Job drawing, mm, ordinate dimensions from the low corner. One solid piece. A direction names the side the tool comes from. Round coordinates to 2 decimals unless told otherwise and drop trailing zeros. Write each loop counter-clockwise with the first axis right and the second up, starting at its lowest first coordinate (ties: lowest second). Pieces come first, ordered by that corner, then holes. Notation, with made-up numbers: M 75,69.5 L 83,69.5 A30 ccw 83,101.5 Z; hole C 59.25,-31.75 d9. An arc over 180 degrees is marked long. Answer as a JSON object with one key per item and string values. Group by question number.
1. Band-saw the part on A-A, the plane x = 64. Write the cut outline in (y, z), plus the area to 3 significant figures.
2. Band-saw the part on D-D, the plane x = 87.1. Write the cut outline in (y, z), plus the area to 3 significant figures.
3. Band-saw the part on B-B, the plane y = 22.1. Write the cut outline in (x, z), plus the area to 3 significant figures.
4. Two-plate mould, pull along X, no slides. Class the marked faces 3 and 4: +X half, -X half, draft (parallel to the pull), parting line (faces both ways), or undercut.
5. Band-saw the part on C-C, the plane z = 3.5. Write the cut outline in (x, y).
6. Which spindle directions (+Z, -Z, +X, -X, +Y, -Y) get a long thin tool onto all of the face, cutting with end or side? Do the marked faces 1 and 2. Say none if no direction does.
7. Drill centre lines: line 1 (Y direction, x = 87.1, z = 4); line 2 (X direction, y = 9.1, z = 3.5); line 3 (X direction, y = 27, z = 2.25). Where is each one in solid material? Low to high. Write a range as from..to.
8. Drop a flat-ended pin along its axis: pin 1 (5 mm diameter, centred on x = 87.1, y = 22.1, fed in from +Z). Give the stop position or say it passes through.
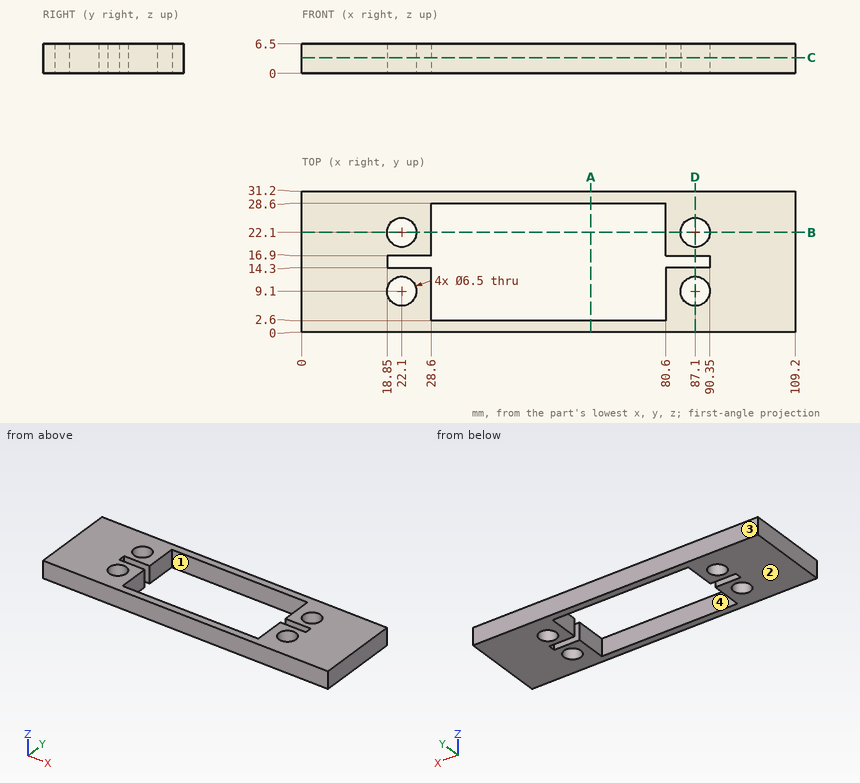
Worked answers:
{
 "1": {"outline": "M 0,0 L 2.6,0 L 2.6,6.5 L 0,6.5 Z; M 28.6,0 L 31.2,0 L 31.2,6.5 L 28.6,6.5 Z", "area": "33.8 mm^2"},
 "2": {"outline": "M 0,0 L 5.85,0 L 5.85,6.5 L 0,6.5 Z; M 12.35,0 L 14.3,0 L 14.3,6.5 L 12.35,6.5 Z; M 16.9,0 L 18.85,0 L 18.85,6.5 L 16.9,6.5 Z; M 25.35,0 L 31.2,0 L 31.2,6.5 L 25.35,6.5 Z", "area": "101 mm^2"},
 "3": {"outline": "M 0,0 L 18.85,0 L 18.85,6.5 L 0,6.5 Z; M 25.35,0 L 28.6,0 L 28.6,6.5 L 25.35,6.5 Z; M 80.6,0 L 83.85,0 L 83.85,6.5 L 80.6,6.5 Z; M 90.35,0 L 109.2,0 L 109.2,6.5 L 90.35,6.5 Z", "area": "287 mm^2"},
 "4": {"face 3": "draft", "face 4": "undercut"},
 "5": {"outline": "M 0,0 L 109.2,0 L 109.2,31.2 L 0,31.2 Z; hole C 22.1,9.1 d6.5; hole M 18.85,14.3 L 28.6,14.3 L 28.6,2.6 L 80.6,2.6 L 80.6,14.3 L 90.35,14.3 L 90.35,16.9 L 80.6,16.9 L 80.6,28.6 L 28.6,28.6 L 28.6,16.9 L 18.85,16.9 Z; hole C 22.1,22.1 d6.5; hole C 87.1,9.1 d6.5; hole C 87.1,22.1 d6.5"},
 "6": {"face 1": "+Z, -Z", "face 2": "-Z, +X, -X, +Y, -Y"},
 "7": {"line 1": "y = 0..5.85, 12.35..14.3, 16.9..18.85, 25.35..31.2", "line 2": "x = 0..18.85, 25.35..28.6, 80.6..83.85, 90.35..109.2", "line 3": "x = 0..28.6, 80.6..109.2"},
 "8": {"pin 1": "passes through"}
}
